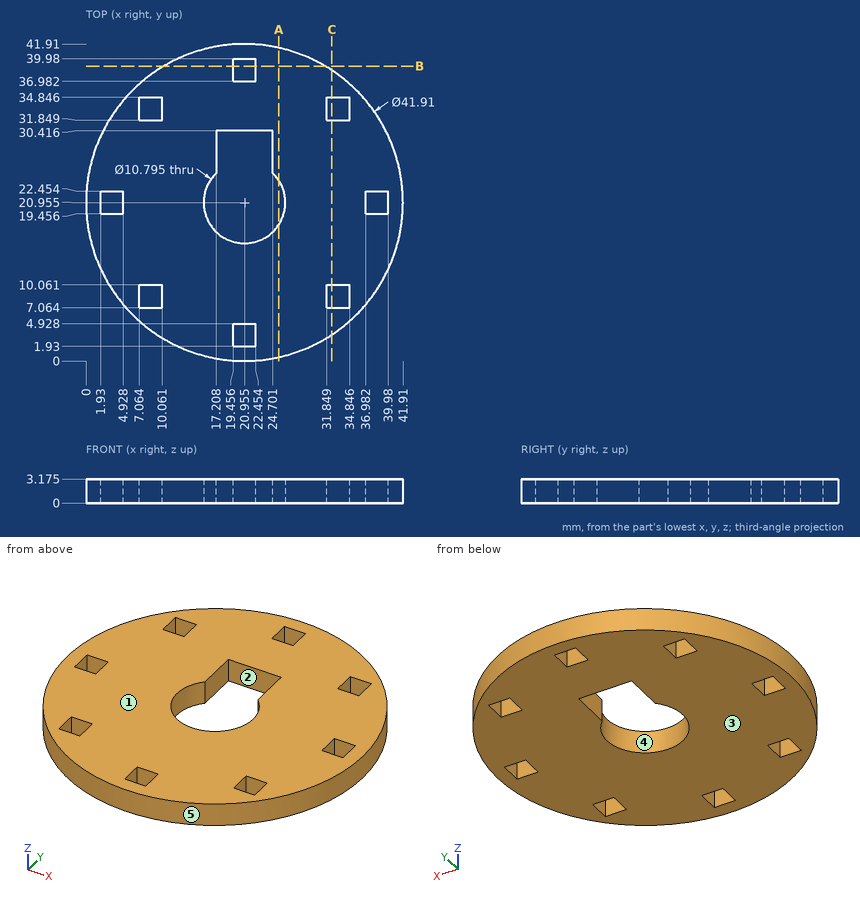
Design review of the part shown in the three views and the two pictorial views. Dimensions are in mm from the part's minimum x, y and z. A direction names the side the tool comes from. Coordinates: 2 decimals unless noted, no trailing zeros. Write each loop counter-clockwise with the first axis right and the second up, starting at its lowest first coordinate (ties: lowest second). Pieces come first, ordered by that corner, then holes.
(1) Add section B-B on y = 39. Give the boundary of the cut face in (x, z) (1 decimal).
(2) For pin 1 Ø1.5 at (x, z) = (21, 1.5) entering from +Y; pin 2 Ø1.6 at (y, z) = (27.5, 1) entering from +X; pin 3 Ø1.5 at (x, z) = (33, 1) entering from +Y (1 decimal), all flat-tipped, find the tip position at first contact; note any pin that passes through.
(3) Add section A-A on x = 25.5. Give the boundary of the cut face in (y, z) (1 decimal), then the cut area to 3 significant figures.
(4) Wall thickness on probe 1 along X at (y, z) = (21.5, 3) (1 decimal); probe 2 along X at (y, z) = (19.5, 1.15); probe 3 along Y at (x, z) = (22, 1.5) (1 decimal): over which ranges is each line inside the solid? List them lowest first.
(5) Tool access review of the marked faces 1 and 2: name each direction out of +Z, -Z, +X, -X, +Y, -Y from which nothing blocks a thin tool from reaching the whole face with its end or side.
(6) The part is to be moulded in two halves that separate along X. For the marked faces 3, 4 and 5, say which applies: +X half, -X half, draft (parallel to the pull), parting line (faces both ways), or undercut.
(7) Add section C-C on x = 32.5. Count the separate pieces of the cut face and the enclosed holes in it.
Answer sheet:
1. outline: (10.3, 0) - (19.5, 0) - (19.5, 3.2) - (10.3, 3.2) - close; (22.5, 0) - (31.6, 0) - (31.6, 3.2) - (22.5, 3.2) - close
2. pin 1: stops at y = 41.91
2. pin 2: stops at x = 41.11
2. pin 3: stops at y = 38.6
3. outline: (0.5, 0) - (18, 0) - (18, 3.2) - (0.5, 3.2) - close; (23.9, 0) - (41.4, 0) - (41.4, 3.2) - (23.9, 3.2) - close
3. area: 111 mm2
4. probe 1: x = 0 to 1.9, 4.9 to 15.6, 26.3 to 37, 40 to 41.9
4. probe 2: x = 0.05 to 1.93, 4.93 to 15.76, 26.15 to 36.98, 39.98 to 41.86
4. probe 3: y = 0 to 1.9, 4.9 to 15.7, 30.4 to 37, 40 to 41.9
5. face 1: +Z, +X, -X, +Y, -Y
5. face 2: +Z, -Z
6. face 3: draft
6. face 4: undercut
6. face 5: parting line
7. separate pieces: 3
7. enclosed holes: 0
